Source: CAD feature listing. Evaluate the final solid. Frame: model axes, mm. Face numbers are marked on the shaded views. A direction names the side the tool comes from. Round coordinates to 2 decimals unless told otherwise and drop trailing zeros. Loops run counter-clockwise (first coordinate to the right, second up) from the corner with the lowest first, then second, coordinate; pieces in that order, holes last. Notation, with made-up numbers: M 14.25,62.25 L 43.25,62.25 A30 cw 43.25,90.25 Z; hole C 9,80.25 d10. An arc over 180 degrees is marked long. One line per item, written item: value.
from build123d import *

# Parameters (mm, degrees)
SKETCH1_R           = 2.75
BOSS_EXTRUDE1_DEPTH = 1.2
SKETCH2_R           = 21.5
BOSS_EXTRUDE2_DEPTH = 12.2
SKETCH3_R           = 15
BOSS_EXTRUDE3_DEPTH = 10
SKETCH5_R           = 12
BOSS_EXTRUDE4_DEPTH = 7
FILLET1_R           = 7


with BuildPart() as part:
    # Sketch1 → Boss-Extrude1 (new body)
    with BuildSketch(Plane(origin=(0, 0, 0), x_dir=(1, 0, 0), z_dir=(0, 1, 0))):
        with BuildLine():
            ThreePointArc((-27.045454545, -4.979295977), (0, -27.5), (27.045454545, -4.979295977))
            ThreePointArc((27.045454545, -4.979295977), (32.5, 0), (27.045454545, 4.979295977))
            ThreePointArc((27.045454545, 4.979295977), (0, 27.5), (-27.045454545, 4.979295977))
            ThreePointArc((-27.045454545, 4.979295977), (-32.5, 0), (-27.045454545, -4.979295977))
        make_face()
        with Locations(Location((-27.5, 0, 0), (0, 0, 270))):
            Circle(SKETCH1_R, mode=Mode.SUBTRACT)
        with Locations(Location((27.5, 0, 0), (0, 0, 270))):
            Circle(SKETCH1_R, mode=Mode.SUBTRACT)
    extrude(amount=BOSS_EXTRUDE1_DEPTH)

    # Sketch2 → Boss-Extrude2 (add)
    with BuildSketch(Plane(origin=(0, 1.2, 0), x_dir=(1, 0, 0), z_dir=(0, 1, 0))):
        with Locations(Location((0, 0, 0), (0, 0, 270))):
            Circle(SKETCH2_R)
    extrude(amount=BOSS_EXTRUDE2_DEPTH)

    # Sketch3 → Boss-Extrude3 (add)
    with BuildSketch(Plane(origin=(0, 13.4, 0), x_dir=(1, 0, 0), z_dir=(0, 1, 0))):
        with Locations(Location((0, 0, 0), (0, 0, 270))):
            Circle(SKETCH3_R)
    extrude(amount=BOSS_EXTRUDE3_DEPTH)

    # Sketch5 → Boss-Extrude4 (add)
    with BuildSketch(Plane(origin=(0, 23.4, 0), x_dir=(1, 0, 0), z_dir=(0, 1, 0))):
        with Locations(Location((0, 0, 0), (0, 0, 270))):
            Circle(SKETCH5_R)
    extrude(amount=BOSS_EXTRUDE4_DEPTH)

    # Fillet1
    fillet1_edges = [part.edges().sort_by_distance(p)[0] for p in [
        (0, 30.4, -12),
    ]]
    fillet(fillet1_edges, radius=FILLET1_R - 0.0001)  # a hair under: the kernel refuses the full size


solid = part.part
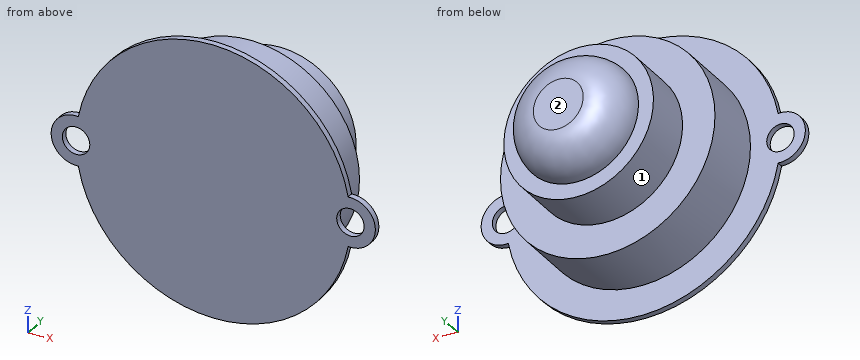
1. Pin query (flat end, axial travel): pin 1 (6 mm diameter, centred on x = 8.5, y = 4.5, fed in from -Z); pin 2 (9 mm diameter, centred on x = 27.5, z = 0, fed in from +Y); pin 3 (10 mm diameter, centred on x = -23.5, y = 5.5, fed in from +Z). Return the tip coordinate at first contact, or that it passes through.
Report:
pin 1: stops at z = -20.78
pin 2: stops at y = 1.2
pin 3: stops at z = 17.82
2. Section query B-B (y = 3). Return the cut outline in (x, z).
Report:
outline: C 0,0 d43
3. Section query C-C (z = 17.5). Return the cut outline in (x, y), and give its area (3 significant figures).
Report:
outline: M -21.21,0 L 21.21,0 L 21.21,1.2 L 12.49,1.2 L 12.49,13.4 L -12.49,13.4 L -12.49,1.2 L -21.21,1.2 Z
area: 356 mm2
4. Section query A-A (z = 0). Count the separate pieces of the cut face and the enclosed holes in it, and give its area (3 significant figures).
Report:
separate pieces: 3
enclosed holes: 0
area: 1,040 mm2
5. Reachability of the marked faces 1 and 2 from +Z, -Z, +X, -X, +Y, -Y: full face, straight path, thin tool, end or side. Return the list, or none.
Report:
face 1: +Y
face 2: +Z, -Z, +X, -X, +Y
6. Section query D-D (y = 19.5). Return the cut outline in (x, z), and give its area (3 significant figures).
Report:
outline: C 0,0 d30
area: 707 mm2
7. Ray query, line 1 (X direction, y = 0.7, z = 0); line 2 (Y direction, x = -6.5, z = 11); line 3 (Y direction, x = 20.5, z = 5). Return the intervals inside material, ascending. Write a range as [from, to].
Report:
line 1: x = [-32.5, -30.25], [-24.75, 24.75], [30.25, 32.5]
line 2: y = [0, 23.4]
line 3: y = [0, 13.4]
